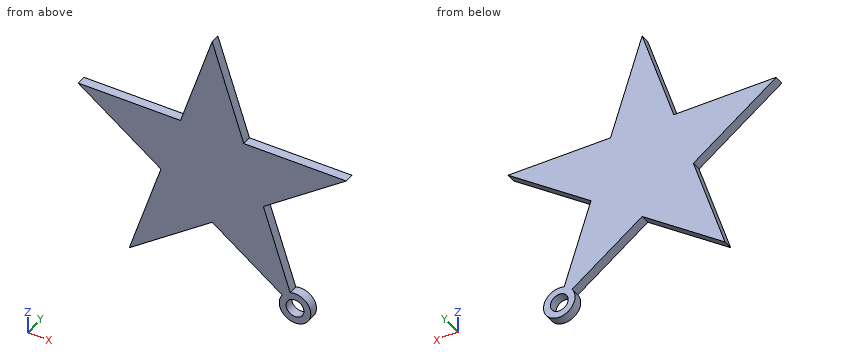
Autodesk Fusion 360 part; units mm, degrees
sketch "草图1" plane through (0, 0, 0) normal (0, 1, 0) x (1, 0, 0)
  line L0 (-52.5144, 0) -> (-26.2572, -80.8114)
  line L1 (0, 0) -> (-26.2572, -80.8114)
  line L2 (0, 0) -> (-68.7423, -49.9442)
  line L3 (-68.7423, -49.9442) -> (16.2279, -49.9442)
  line L4 (16.2279, -49.9442) -> (-52.5144, 0)
  circle A0 centre (0, 0) radius 5
  circle A1 centre (0, 0) radius 2.8284
  point P0 (-26.2572, -36.14)
extrude "拉伸1" add sketch "草图1" along normal blind 3 contours L0 L2 L4 | L0 L1 L2 L3 L4 | L0 L2 L3 | L1 L2 L4 A0 | L0 L1 L3 | L1 L2 A0 A1 | L1 L2 A0 A1 | L1 L3 L4
Check sheet for the modelled part. Datum: model origin and axes. Units: mm. Round coordinates to 2 decimals unless told otherwise and drop trailing zeros. Loops run counter-clockwise (first coordinate to the right, second up) from the corner with the lowest first, then second, coordinate; pieces in that order, holes last.
1. Sectioned sample at A-A on y = 1.4. Record the boundary of the cut face in (x, z), and give its area (3 significant figures).
2. Sectioned sample at B-B on x = -9. Record the boundary of the cut face in (y, z), and give its area (3 significant figures).
3. Sectioned sample at C-C on x = 0. Record the boundary of the cut face in (y, z), and give its area (3 significant figures).
4. Scan lines: probe 1 along Z at (x, y) = (0, 1.65); probe 2 along X at (y, z) = (0.9, 18); probe 3 along X at (y, z) = (2, 4.5). Record each from-to range of solid material in increasing order.
5. Sectioned sample at D-D on z = 34. Record the boundary of the cut face in (x, y).
6. Gauge pin test, flat ends, axial feed: pin 1 Ø1.5 at (x, y) = (-56, 2.5) entering from -Z; pin 2 Ø0.9 at (x, y) = (-7.5, 1) entering from +Z; pin 3 Ø6 at (x, z) = (-38, 59.5) entering from -Y. Record the tip position at first contact, or that the pin passes through.
Recorded:
1. outline: (-68.74, 49.94) - (-42.49, 30.87) - (-52.51, 0) - (-26.26, 19.08) - (-4.05, 2.94) arc R5 ccw (long way) to (-1.55, 4.76) - (-10.03, 30.87) - (16.23, 49.94) - (-16.23, 49.94) - (-26.26, 80.81) - (-36.29, 49.94) - close; hole circle Ø5.66 at (0, 0)
1. area: 2,290 mm2
2. outline: (0, 6.54) - (3, 6.54) - (3, 27.7) - (0, 27.7) - close; (0, 31.62) - (3, 31.62) - (3, 49.94) - (0, 49.94) - close
2. area: 118 mm2
3. outline: (0, -5) - (3, -5) - (3, -2.83) - (0, -2.83) - close; (0, 2.83) - (3, 2.83) - (3, 5) - (0, 5) - close; (0, 38.15) - (3, 38.15) - (3, 49.94) - (0, 49.94) - close
3. area: 48.4 mm2
4. probe 1: z = -5 to -2.83, 2.83 to 5, 38.15 to 49.94
4. probe 2: x = -46.67 to -27.74, -24.77 to -5.85
4. probe 3: x = -51.05 to -46.32, -6.19 to 2.18
5. outline: (-46.8, 0) - (-5.72, 0) - (-5.72, 3) - (-46.8, 3) - close
6. pin 1: stops at z = 40.14
6. pin 2: stops at z = 49.94
6. pin 3: passes through
